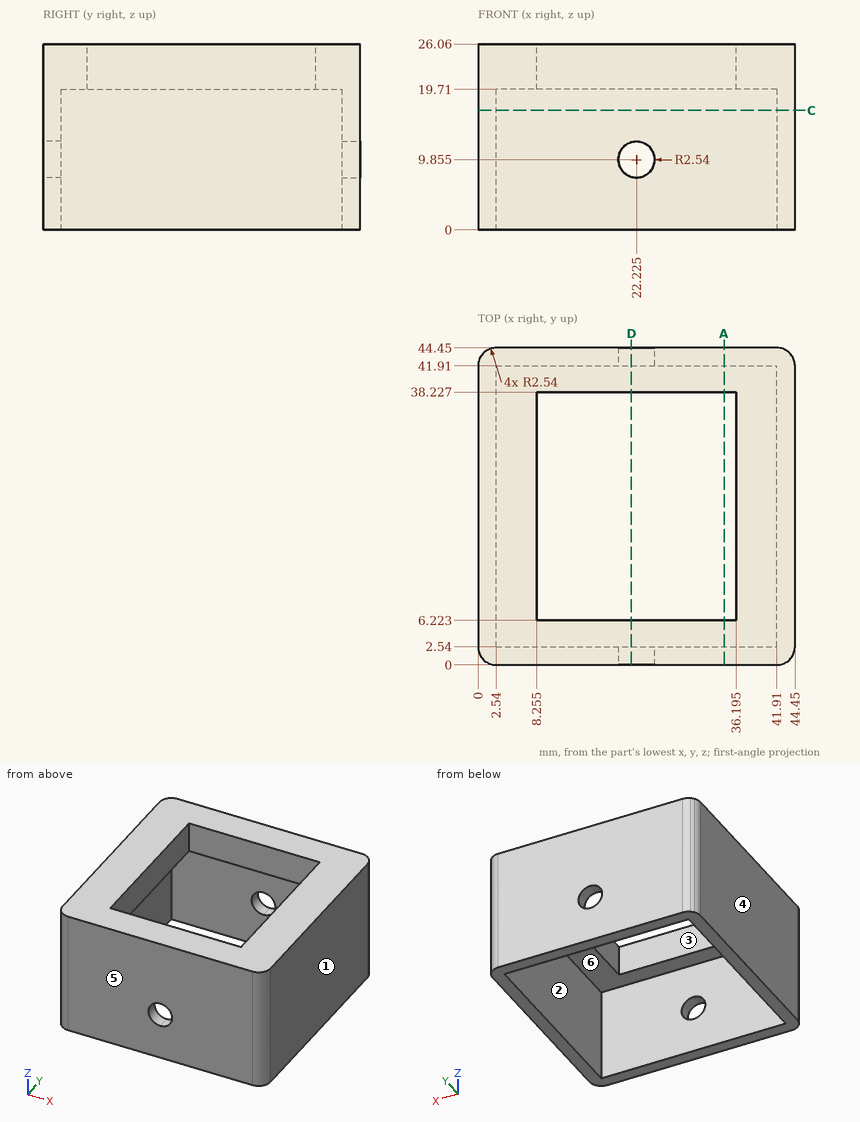
Job drawing, mm, ordinate dimensions from the low corner. One solid piece. A direction names the side the tool comes from. Give positions to 0.01 mm unless a question says otherwise; leave off trailing zeros. Order: outer loops, then holes, each group sorted by start corner. A loop starts at its lowest first (then second) coordinate and runs counter-clockwise, first axis right, second up. Notation, with made-up numbers: (56, 12) - (68, 12) arc R23 cw to (68, 43) - close; hole circle Ø3 at (-3, -19). An arc over 180 degrees is marked (long way). Answer in a Markdown table with one row per item.
1. Saw through at C-C, the plane z = 16.75. Give the cut face in (x, y).
Data:
| item | result |
|---|---|
| outline | (0, 2.54) arc R2.54 ccw to (2.54, 0) - (41.91, 0) arc R2.54 ccw to (44.45, 2.54) - (44.45, 41.91) arc R2.54 ccw to (41.91, 44.45) - (2.54, 44.45) arc R2.54 ccw to (0, 41.91) - close; hole (2.54, 2.54) - (41.91, 2.54) - (41.91, 41.91) - (2.54, 41.91) - close |
2. Saw through at A-A, the plane x = 34.5. Give the cut face in (y, z), plus the area to 3 significant figures.
Data:
| item | result |
|---|---|
| outline | (0, 0) - (2.54, 0) - (2.54, 19.71) - (6.22, 19.71) - (6.22, 26.06) - (0, 26.06) - close; (38.23, 19.71) - (41.91, 19.71) - (41.91, 0) - (44.45, 0) - (44.45, 26.06) - (38.23, 26.06) - close |
| area | 179 mm² |
3. Probe probe 1 along Y at (x, z) = (39, 2.5); probe 2 along Y at (x, z) = (20, 25). List the from-to ranges inside material, lowest first. Write a range as [from, to].
Data:
| item | result |
|---|---|
| probe 1 | y = [0, 2.54], [41.91, 44.45] |
| probe 2 | y = [0, 6.22], [38.23, 44.45] |
4. Saw through at D-D, the plane x = 21.5. Give the cut face in (y, z).
Data:
| item | result |
|---|---|
| outline | (0, 0) - (2.54, 0) - (2.54, 7.42) - (0, 7.42) - close; (0, 12.29) - (2.54, 12.29) - (2.54, 19.71) - (6.22, 19.71) - (6.22, 26.06) - (0, 26.06) - close; (38.23, 19.71) - (41.91, 19.71) - (41.91, 12.29) - (44.45, 12.29) - (44.45, 26.06) - (38.23, 26.06) - close; (41.91, 0) - (44.45, 0) - (44.45, 7.42) - (41.91, 7.42) - close |
5. Pull direction Y, two halves, no side cores. Call the marked faces 4, 5 and 6: pulls with the +Y half, pulls with the -Y half, needs draft (parallel to the pull), parting line crosses it, or undercut.
Data:
| item | result |
|---|---|
| face 4 | needs draft |
| face 5 | pulls with the -Y half |
| face 6 | undercut |
6. Tool access for the marked faces 1, 2 and 3: list every direction of +Z, -Z, +X, -X, +Y, -Y with a clear straight run to the whole face (end or side of a thin tool).
Data:
| item | result |
|---|---|
| face 1 | +Z, -Z, +X, +Y, -Y |
| face 2 | -Z |
| face 3 | +Z, -Z |
